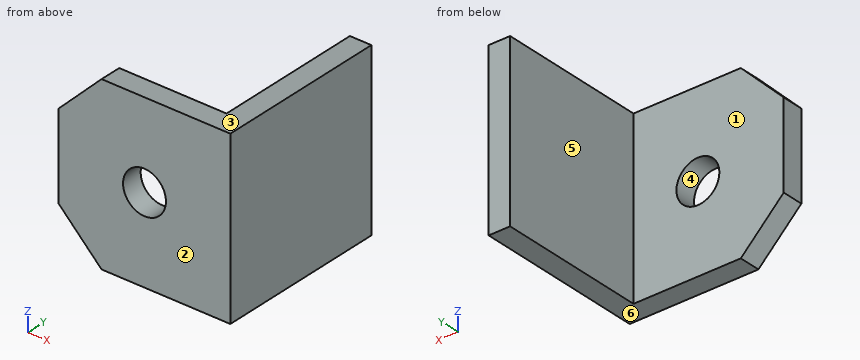
from build123d import *

# Parameters (mm, degrees)
EXTRUDE_THIN1_DEPTH = 40
CHAMFER1_SIZE       = 10
SKETCH2_R           = 5
CUT_EXTRUDE1_DEPTH  = 10


with BuildPart() as part:
    # Sketch1 → Extrude-Thin1 (new body)
    with BuildSketch(Plane.XY):
        Polygon((-40, 0), (0, 0), (0, 40), (-5, 40), (-5, 5), (-40, 5), align=None)
    extrude(amount=EXTRUDE_THIN1_DEPTH)

    # Chamfer1
    chamfer1_edges = [part.edges().sort_by_distance(p)[0] for p in [
        (-40, 2.5, 40),
        (-40, 2.5, 0),
    ]]
    chamfer(chamfer1_edges, length=CHAMFER1_SIZE)

    # Sketch2 → Cut-Extrude1 (cut)
    with BuildSketch(Plane(origin=(0, 5, 0), x_dir=(1, 0, 0), z_dir=(0, 1, 0))):
        with Locations(Location((-20, -20, 0), (0, 0, 270))):
            Circle(SKETCH2_R)
    extrude(amount=-CUT_EXTRUDE1_DEPTH, mode=Mode.SUBTRACT)


solid = part.part
Design review of the part built by this model. Coordinates are the model's own, in mm. Face numbers are marked on the shaded views. A direction names the side the tool comes from. Round coordinates to 2 decimals unless told otherwise and drop trailing zeros. Write each loop counter-clockwise with the first axis right and the second up, starting at its lowest first coordinate (ties: lowest second). Pieces come first, ordered by that corner, then holes.
Item 1: Consider section C-C on z = 31.5. Give the boundary of the cut face in (x, y).
Item 2: Consider section B-B on x = -20. Give the boundary of the cut face in (y, z).
Item 3: Draft analysis for pull direction Z (two halves, no side actions). For the marked faces 3, 4, 5 and 6, state which applies: released by +Z, released by -Z, zero draft, split by the parting line, or undercut.
Item 4: Consider section A-A on z = 20. Give the boundary of the cut face in (x, y).
Item 5: Consider section D-D on x = -34.5. Give the boundary of the cut face in (y, z).
Item 6: Wall thickness on L1, parallel to X at y = 3.1, z = 20; L2, parallel to X at y = 16, z = 14; L3, parallel to Y at x = -30, z = 16: over which ranges is each line inside the solid? List them lowest first.
Item 7: For pin 1 Ø13 at (x, z) = (-20, 20) entering from +Y; pin 2 Ø5 at (x, z) = (-19, 19.5) entering from -Y; pin 3 Ø17.5 at (y, z) = (23.5, 23.5) entering from -X, all flat-tipped, find the tip position at first contact; note any pin that passes through.
Item 8: For the marked faces 1 and 2, list the 3-axis set-ups (+Z, -Z, +X, -X, +Y, -Y) from which the entire face can be reached by the end or side of a thin tool; tool diameter is ignored.
Check values:
1. outline: (-38.5, 0) - (0, 0) - (0, 40) - (-5, 40) - (-5, 5) - (-38.5, 5) - close
2. outline: (0, 0) - (5, 0) - (5, 15) - (0, 15) - close; (0, 25) - (5, 25) - (5, 40) - (0, 40) - close
3. face 3: released by +Z
3. face 4: undercut
3. face 5: zero draft
3. face 6: released by -Z
4. outline: (-40, 0) - (-25, 0) - (-25, 5) - (-40, 5) - close; (-15, 0) - (0, 0) - (0, 40) - (-5, 40) - (-5, 5) - (-15, 5) - close
5. outline: (0, 4.5) - (5, 4.5) - (5, 35.5) - (0, 35.5) - close
6. L1: x = -40 to -25, -15 to 0
6. L2: x = -5 to 0
6. L3: y = 0 to 5
7. pin 1: stops at y = 5
7. pin 2: passes through
7. pin 3: stops at x = -5
8. face 1: +Z, -Z, -X, +Y
8. face 2: +Z, -Z, +X, -X, -Y
